```python
from build123d import *

# Parameters (mm, degrees)
BR_EXTRUDE_DEPTH      = 320
BR_EXTRUDE_DEPTH_BACK = 320


with BuildPart() as part:
    # Sketch2 → BR_Extrude (new body, two sides)
    with BuildSketch(Plane(origin=(0, 0, 0), x_dir=(0, 0, -1), z_dir=(1, 0, 0))) as br_extrude_sk:
        with BuildLine():
            Line((-10.05, 11.464213562), (-10.05, 14))
            Line((-10.05, 14), (-5, 14))
            Line((-5, 14), (-5, 18.5))
            Line((-5, 18.5), (-5.8, 18.5))
            Line((-5.8, 18.5), (-5.8, 20))
            Line((-5.8, 20), (-17, 20))
            ThreePointArc((-17, 20), (-19.121320344, 19.121320344), (-20, 17))
            Line((-20, 17), (-20, 5.8))
            Line((-20, 5.8), (-18.5, 5.8))
            Line((-18.5, 5.8), (-18.5, 5))
            Line((-18.5, 5), (-14, 5))
            Line((-14, 5), (-14, 10.05))
            Line((-14, 10.05), (-11.464213562, 10.05))
            Line((-11.464213562, 10.05), (-7.5, 6.085786438))
            Line((-7.5, 6.085786438), (-7.5, -6.085786438))
            Line((-7.5, -6.085786438), (-11.464213562, -10.05))
            Line((-11.464213562, -10.05), (-14, -10.05))
            Line((-14, -10.05), (-14, -5))
            Line((-14, -5), (-18.5, -5))
            Line((-18.5, -5), (-18.5, -5.8))
            Line((-18.5, -5.8), (-20, -5.8))
            Line((-20, -5.8), (-20, -17))
            ThreePointArc((-20, -17), (-19.121320344, -19.121320344), (-17, -20))
            Line((-17, -20), (-5.8, -20))
            Line((-5.8, -20), (-5.8, -18.5))
            Line((-5.8, -18.5), (-5, -18.5))
            Line((-5, -18.5), (-5, -14))
            Line((-5, -14), (-10.05, -14))
            Line((-10.05, -14), (-10.05, -11.464213562))
            Line((-10.05, -11.464213562), (-6.085786438, -7.5))
            Line((-6.085786438, -7.5), (6.085786438, -7.5))
            Line((6.085786438, -7.5), (10.05, -11.464213562))
            Line((10.05, -11.464213562), (10.05, -14))
            Line((10.05, -14), (5, -14))
            Line((5, -14), (5, -18.5))
            Line((5, -18.5), (5.8, -18.5))
            Line((5.8, -18.5), (5.8, -20))
            Line((5.8, -20), (17, -20))
            ThreePointArc((17, -20), (19.121320344, -19.121320344), (20, -17))
            Line((20, -17), (20, -5.8))
            Line((20, -5.8), (18.5, -5.8))
            Line((18.5, -5.8), (18.5, -5))
            Line((18.5, -5), (14, -5))
            Line((14, -5), (14, -10.05))
            Line((14, -10.05), (11.464213562, -10.05))
            Line((11.464213562, -10.05), (7.5, -6.085786438))
            Line((7.5, -6.085786438), (7.5, 6.085786438))
            Line((7.5, 6.085786438), (11.464213562, 10.05))
            Line((11.464213562, 10.05), (14, 10.05))
            Line((14, 10.05), (14, 5))
            Line((14, 5), (18.5, 5))
            Line((18.5, 5), (18.5, 5.8))
            Line((18.5, 5.8), (20, 5.8))
            Line((20, 5.8), (20, 17))
            ThreePointArc((20, 17), (19.121320344, 19.121320344), (17, 20))
            Line((17, 20), (5.8, 20))
            Line((5.8, 20), (5.8, 18.5))
            Line((5.8, 18.5), (5, 18.5))
            Line((5, 18.5), (5, 14))
            Line((5, 14), (10.05, 14))
            Line((10.05, 14), (10.05, 11.464213562))
            Line((10.05, 11.464213562), (6.085786438, 7.5))
            Line((6.085786438, 7.5), (-6.085786438, 7.5))
            Line((-6.085786438, 7.5), (-10.05, 11.464213562))
        make_face()
        with BuildLine():
            Line((8, 15.5), (8, 18.5))
            Line((8, 18.5), (14.5, 18.5))
            Line((14.5, 18.5), (14.5, 17.25))
            ThreePointArc((14.5, 17.25), (16.444543648, 16.444543648), (17.25, 14.5))
            Line((17.25, 14.5), (18.5, 14.5))
            Line((18.5, 14.5), (18.5, 8))
            Line((18.5, 8), (15.5, 8))
            Line((15.5, 8), (15.5, 11.75))
            Line((15.5, 11.75), (14.5, 11.75))
            ThreePointArc((14.5, 11.75), (12.555456352, 12.555456352), (11.75, 14.5))
            Line((11.75, 14.5), (11.75, 15.5))
            Line((11.75, 15.5), (8, 15.5))
        make_face(mode=Mode.SUBTRACT)
        with BuildLine():
            Line((8, -15.5), (11.75, -15.5))
            Line((11.75, -15.5), (11.75, -14.5))
            ThreePointArc((11.75, -14.5), (12.555456352, -12.555456352), (14.5, -11.75))
            Line((14.5, -11.75), (15.5, -11.75))
            Line((15.5, -11.75), (15.5, -8))
            Line((15.5, -8), (18.5, -8))
            Line((18.5, -8), (18.5, -14.5))
            Line((18.5, -14.5), (17.25, -14.5))
            ThreePointArc((17.25, -14.5), (16.444543648, -16.444543648), (14.5, -17.25))
            Line((14.5, -17.25), (14.5, -18.5))
            Line((14.5, -18.5), (8, -18.5))
            Line((8, -18.5), (8, -15.5))
        make_face(mode=Mode.SUBTRACT)
        with BuildLine():
            Line((-15.5, 8), (-18.5, 8))
            Line((-18.5, 8), (-18.5, 14.5))
            Line((-18.5, 14.5), (-17.25, 14.5))
            ThreePointArc((-17.25, 14.5), (-16.444543648, 16.444543648), (-14.5, 17.25))
            Line((-14.5, 17.25), (-14.5, 18.5))
            Line((-14.5, 18.5), (-8, 18.5))
            Line((-8, 18.5), (-8, 15.5))
            Line((-8, 15.5), (-11.75, 15.5))
            Line((-11.75, 15.5), (-11.75, 14.5))
            ThreePointArc((-11.75, 14.5), (-12.555456352, 12.555456352), (-14.5, 11.75))
            Line((-14.5, 11.75), (-15.5, 11.75))
            Line((-15.5, 11.75), (-15.5, 8))
        make_face(mode=Mode.SUBTRACT)
        with BuildLine():
            Line((-11.75, -14.5), (-11.75, -15.5))
            Line((-11.75, -15.5), (-8, -15.5))
            Line((-8, -15.5), (-8, -18.5))
            Line((-8, -18.5), (-14.5, -18.5))
            Line((-14.5, -18.5), (-14.5, -17.25))
            ThreePointArc((-14.5, -17.25), (-16.444543648, -16.444543648), (-17.25, -14.5))
            Line((-17.25, -14.5), (-18.5, -14.5))
            Line((-18.5, -14.5), (-18.5, -8))
            Line((-18.5, -8), (-15.5, -8))
            Line((-15.5, -8), (-15.5, -11.75))
            Line((-15.5, -11.75), (-14.5, -11.75))
            ThreePointArc((-14.5, -11.75), (-12.555456352, -12.555456352), (-11.75, -14.5))
        make_face(mode=Mode.SUBTRACT)
        with BuildLine():
            Line((-5.2, -5.2), (-5.2, -2.26102435))
            Line((-5.2, -2.26102435), (-4.585300372, -1.993745345))
            ThreePointArc((-4.585300372, -1.993745345), (-5, 0), (-4.585300372, 1.993745345))
            Line((-4.585300372, 1.993745345), (-5.2, 2.26102435))
            Line((-5.2, 2.26102435), (-5.2, 5.2))
            Line((-5.2, 5.2), (-2.26102435, 5.2))
            Line((-2.26102435, 5.2), (-1.993745345, 4.585300372))
            ThreePointArc((-1.993745345, 4.585300372), (0, 5), (1.993745345, 4.585300372))
            Line((1.993745345, 4.585300372), (2.26102435, 5.2))
            Line((2.26102435, 5.2), (5.2, 5.2))
            Line((5.2, 5.2), (5.2, 2.26102435))
            Line((5.2, 2.26102435), (4.585300372, 1.993745345))
            ThreePointArc((4.585300372, 1.993745345), (5, 0), (4.585300372, -1.993745345))
            Line((4.585300372, -1.993745345), (5.2, -2.26102435))
            Line((5.2, -2.26102435), (5.2, -5.2))
            Line((5.2, -5.2), (2.26102435, -5.2))
            Line((2.26102435, -5.2), (1.993745345, -4.585300372))
            ThreePointArc((1.993745345, -4.585300372), (0, -5), (-1.993745345, -4.585300372))
            Line((-1.993745345, -4.585300372), (-2.26102435, -5.2))
            Line((-2.26102435, -5.2), (-5.2, -5.2))
        make_face(mode=Mode.SUBTRACT)
    extrude(amount=BR_EXTRUDE_DEPTH)
    extrude(br_extrude_sk.sketch, amount=-BR_EXTRUDE_DEPTH_BACK)


solid = part.part
```
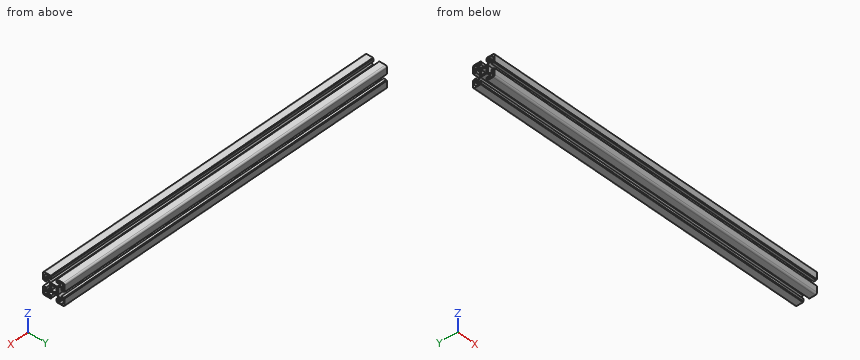
Input: part model. Units: mm. Frame: model coordinates. Give positions to 0.01 mm unless a question says otherwise; leave off trailing zeros.
1. Cut plane A-A (x = -76). State how many separate pieces and enclosed holes the cut face has, and give its area (3 significant figures).
Computed:
separate pieces: 1
enclosed holes: 5
area: 555 mm2
2. Pin query (flat end, axial travel): pin 1 Ø1.6 at (x, y) = (-1, 19.5) entering from -Z; pin 2 Ø2.5 at (x, z) = (159, -4.5) entering from -Y. Return the tip coordinate at first contact, or that it passes through.
Computed:
pin 1: stops at z = -19.47
pin 2: stops at y = -18.5
3. Line query: probe 1 along Y at (x, z) = (-137, 11.5); probe 2 along Y at (x, z) = (279, 4.5); probe 3 along Y at (x, z) = (-185, -6). Output: solid intervals per line, ascending.
Computed:
probe 1: y = -20 to -18.5, -15.5 to -10.05, 10.05 to 15.5, 18.5 to 20
probe 2: y = -7.5 to -5.2, 5.2 to 7.5
probe 3: y = -20 to -14, -7.5 to 7.5, 14 to 20
